Source: CAD feature listing. Evaluate the final solid. Frame: model axes, mm. Give positions to 0.01 mm unless a question says otherwise; leave off trailing zeros. Order: outer loops, then holes, each group sorted by start corner. A loop starts at its lowest first (then second) coordinate and runs counter-clockwise, first axis right, second up.
1) Section A-A, the plane y = 8. Return loops of the section in (x, z).
2) Material intervals for line 1 (Z direction, x = 0.1, y = 7.5); line 2 (Z direction, x = -0.95, y = 19); line 3 (Z direction, x = -1.05, y = 37), sorted ascending.
3) Section B-B, the plane x = 0.8. Return loops of the section in (y, z), plus the area to 3 significant figures.
4) First-contact query: P1, Ø0.9, axis at x = 0, y = 6.5, coming from the +Z side. Flat tip, straight axial feed; report the tip coordinate or a pass-through.
Autodesk Inventor part; units mm, degrees
ref_plane "YZ Plane" through (0, 0, 0) normal (1, 0, 0) x (0, 1, 0)
ref_plane "XZ Plane" through (0, 0, 0) normal (0, 1, 0) x (-1, 0, 0)
ref_plane "XY Plane" through (0, 0, 0) normal (0, 0, 1) x (1, 0, 0)
sketch "Sketch2" plane through (0, 0, 0) normal (0, 1, 0) x (-1, 0, 0)
  line L0 (-1.5, -198.6195) -> (1.5, -198.6195)
  line L1 (1.5, -198.6195) -> (1.5, 198.6195)
  line L2 (1.5, 198.6195) -> (-1.5, 198.6195)
  line L3 (-1.5, 198.6195) -> (-1.5, -198.6195)
  line L4 (-1.5, -198.6195) -> (1.5, 198.6195) construction
  line L5 (1.5, -198.6195) -> (-1.5, 198.6195) construction
  point P0 (0, 0)
  dimension "d0" = 3
  dimension "d1" = 397.239
extrude "Extrusion1" add sketch "Sketch2" along normal blind 40
sketch "Sketch3" plane through (1.5, 0, 198.6195) normal (1, 0, 0) x (0, 0, -1)
  line L0 (397.239, 0) -> (0, 0)
  line L1 (68, 0) -> (82, 0)
  line L2 (82, 0) -> (82, 14)
  line L3 (68, 14) -> (68, 0)
  arc A0 (82, 14) -> (68, 14) centre (75, 14) ccw
  arc A1 (68, 14) -> (82, 14) centre (75, 14) ccw construction
  line L4 (0, 0) -> (0, 40)
  point P0 (198.6195, 0)
  dimension "d4" = 14
  dimension "d5" = 14
  dimension "d6" = 14
  dimension "d9" = 75
extrude "Extrusion2" cut sketch "Sketch3" against normal through all
sketch "Sketch4" plane through (1.5, 0, -198.6195) normal (1, 0, 0) x (0, 0, -1)
  line L0 (-329.239, 0) -> (-397.239, 0)
  line L1 (-397.239, 0) -> (-397.239, 40)
  line L2 (-397.239, 0) -> (-397.239, 40)
  line L3 (-397.239, 40) -> (-390.1859, 40)
  line L4 (-397.239, 40) -> (0, 40)
  line L5 (-397.239, 0) -> (-390.1859, 40)
  point P0 (-198.6195, 0)
  dimension "d10" = 10
extrude "Extrusion3" cut sketch "Sketch4" against normal through all
properties part number "wall-inner-plunger"
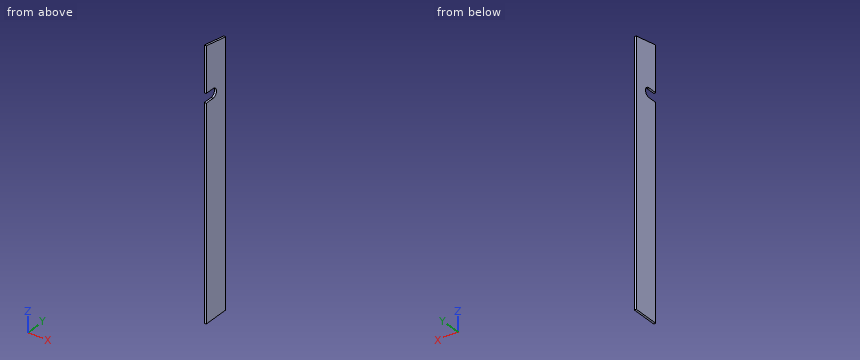
From the geometry:
1. outline: (-1.5, -198.62) - (1.5, -198.62) - (1.5, 116.62) - (-1.5, 116.62) - close; (-1.5, 130.62) - (1.5, 130.62) - (1.5, 197.21) - (-1.5, 197.21) - close
2. line 1: z = -198.62 to 116.62, 130.62 to 197.3
2. line 2: z = -198.62 to 118.72, 128.52 to 195.27
2. line 3: z = -198.62 to 192.1
3. outline: (0, -198.62) - (40, -198.62) - (40, 191.57) - (0, 198.62) - (0, 130.62) - (14, 130.62) arc R7 cw to (14, 116.62) - (0, 116.62) - close
3. area: 15,500 mm2
4. P1: stops at z = 197.55
